Design review of the part built by this model. Coordinates are the model's own, in mm. Face numbers are marked on the shaded views. Coordinates: 2 decimals unless noted, no trailing zeros. Loops run counter-clockwise (first coordinate to the right, second up) from the corner with the lowest first, then second, coordinate; pieces in that order, holes last. Notation, with made-up numbers: (76, -6.75) - (88, -6.75) arc R16 cw to (88, 1.25) - close; hole circle Ø3 at (63.5, 12.25). An arc over 180 degrees is marked (long way). One line per question, with ' | ' between items.
from build123d import *

# Parameters (mm, degrees)
SKETCH1_R               = 6.5
BOSS_EXTRUDE1_DEPTH     = 40
SKETCH2_R               = 7.5
BOSS_EXTRUDE2_DEPTH     = 2
BOSS_EXTRUDE3_DEPTH     = 10
CUT_EXTRUDE1_DEPTH      = 55.004629431
CUT_EXTRUDE1_DEPTH_BACK = 55.004629431
CUT_EXTRUDE2_DEPTH      = 54.619586107
CUT_EXTRUDE2_DEPTH_BACK = 54.619586107
SKETCH5_R               = 0.75
CUT_EXTRUDE3_DEPTH      = 30


with BuildPart() as part:
    # Sketch1 → Boss-Extrude1 (new body)
    with BuildSketch(Plane(origin=(0, 0, 0), x_dir=(0, 0, -1), z_dir=(1, 0, 0))):
        Circle(SKETCH1_R)
    extrude(amount=BOSS_EXTRUDE1_DEPTH)

    # Sketch2 → Boss-Extrude2 (add)
    with BuildSketch(Plane(origin=(40, 0, 0), x_dir=(0, 0, -1), z_dir=(1, 0, 0))):
        Circle(SKETCH2_R)
    extrude(amount=BOSS_EXTRUDE2_DEPTH)

    # Sketch3 → Boss-Extrude3 (add)
    with BuildSketch(Plane(origin=(42, 0, 0), x_dir=(0, 0, -1), z_dir=(1, 0, 0))):
        with BuildLine():
            ThreePointArc((5.590169944, 5), (0, 7.5), (-5.590169944, 5))
            Line((-5.590169944, 5), (-4.898979486, 5))
            Line((-4.898979486, 5), (4.898979486, 5))
            Line((4.898979486, 5), (5.590169944, 5))
        make_face()
        with BuildLine():
            Line((-4.898979486, -5), (-5.590169944, -5))
            ThreePointArc((-5.590169944, -5), (0, -7.5), (5.590169944, -5))
            Line((5.590169944, -5), (4.898979486, -5))
            Line((4.898979486, -5), (-4.898979486, -5))
        make_face()
    extrude(amount=BOSS_EXTRUDE3_DEPTH)

    # Sketch4 → Cut-Extrude1 (cut, two sides: drawn at the far end of the back side and taken through both)
    with BuildSketch(Plane.XZ.offset(-5).offset(-CUT_EXTRUDE1_DEPTH_BACK)):
        with BuildLine():
            Line((42, 5.590169944), (52, 5.590169944))
            Line((52, 5.590169944), (52, -5.590169944))
            Line((52, -5.590169944), (42, -5.590169944))
            Line((42, -5.590169944), (44.640400827, -3.590169944))
            Line((44.640400827, -3.590169944), (47.640400827, -3.590169944))
            add(Edge.make_bspline(
                [(47.640400827, -3.590169944), (50.280133609, -2.393446629), (52.919866391, 0), (50.280133609, 2.393446629), (47.640400827, 3.590169944)],
                knots=[0.178885438, 0.178885438, 0.178885438, 0.178885438, 0.5, 0.821114562, 0.821114562, 0.821114562, 0.821114562], degree=3))
            Line((47.640400827, 3.590169944), (44.640400827, 3.590169944))
            Line((44.640400827, 3.590169944), (42, 5.590169944))
        make_face()
    extrude(amount=CUT_EXTRUDE1_DEPTH + CUT_EXTRUDE1_DEPTH_BACK, mode=Mode.SUBTRACT)

    # Sketch5 → Cut-Extrude2 (cut, two sides: drawn at the far end of the back side and taken through both)
    with BuildSketch(Plane.XZ.offset(-5).offset(-CUT_EXTRUDE2_DEPTH_BACK)):
        with Locations(Location((49, 0, 0), (0, 0, 270))):
            Circle(SKETCH5_R)
    extrude(amount=CUT_EXTRUDE2_DEPTH + CUT_EXTRUDE2_DEPTH_BACK, mode=Mode.SUBTRACT)

    # Sketch6 → Cut-Extrude3 (cut)
    with BuildSketch(Plane.ZY):
        with BuildLine():
            Line((4, -0.5), (4.974937186, -0.5))
            ThreePointArc((4.974937186, -0.5), (3.535533906, -3.535533906), (0.5, -4.974937186))
            Line((0.5, -4.974937186), (0.5, -4))
            Line((0.5, -4), (-0.5, -4))
            Line((-0.5, -4), (-0.5, -4.974937186))
            ThreePointArc((-0.5, -4.974937186), (-3.535533906, -3.535533906), (-4.974937186, -0.5))
            Line((-4.974937186, -0.5), (-4, -0.5))
            Line((-4, -0.5), (-4, 0.5))
            Line((-4, 0.5), (-4.974937186, 0.5))
            ThreePointArc((-4.974937186, 0.5), (-3.535533906, 3.535533906), (-0.5, 4.974937186))
            Line((-0.5, 4.974937186), (-0.5, 4))
            Line((-0.5, 4), (0.5, 4))
            Line((0.5, 4), (0.5, 4.974937186))
            ThreePointArc((0.5, 4.974937186), (3.535533906, 3.535533906), (4.974937186, 0.5))
            Line((4.974937186, 0.5), (4, 0.5))
            Line((4, 0.5), (4, -0.5))
        make_face()
    extrude(amount=-CUT_EXTRUDE3_DEPTH, mode=Mode.SUBTRACT)


solid = part.part
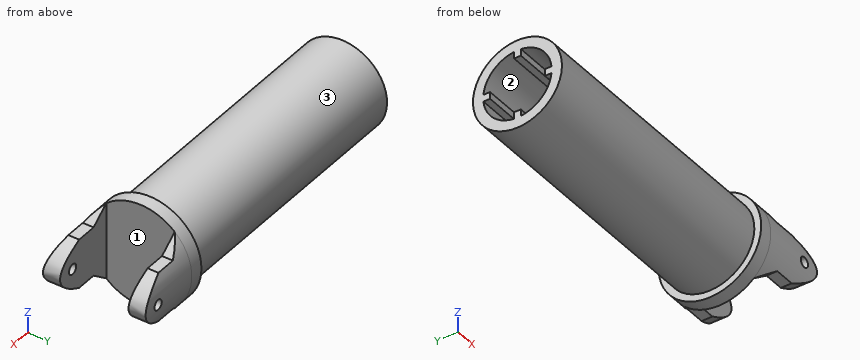
Q1. Take a section at C-C (x = 9). Give the boundary of the cut face in (y, z), plus the area to 3 significant figures.
Returned:
outline: circle Ø13 at (0, 0); hole (-4.97, -0.5) arc R5 ccw to (-0.5, -4.97) - (-0.5, -4) - (0.5, -4) - (0.5, -4.97) arc R5 ccw to (4.97, -0.5) - (4, -0.5) - (4, 0.5) - (4.97, 0.5) arc R5 ccw to (0.5, 4.97) - (0.5, 4) - (-0.5, 4) - (-0.5, 4.97) arc R5 ccw to (-4.97, 0.5) - (-4, 0.5) - (-4, -0.5) - close | area: 58.2 mm²
Q2. To check wall thickness, follow line 1 along X through (y, z) = (5.6, 0); line 2 along X through (y, z) = (6.75, 0); line 3 along X through (y, z) = (-1.75, 4.5). State the ranges of each line that lie inside material, in increasing order.
Returned:
line 1: x = 0 to 48.25, 49.75 to 51.6 | line 2: x = 40 to 48.25, 49.75 to 51.6 | line 3: x = 30 to 42
Q3. Take a section at B-B (y = 0). Give the boundary of the cut face in (x, z), plus the area to 3 significant figures.
Returned:
outline: (0, -6.5) - (40, -6.5) - (40, -7.5) - (42, -7.5) - (42, 7.5) - (40, 7.5) - (40, 6.5) - (0, 6.5) - (0, 4) - (30, 4) - (30, -4) - (0, -4) - close | area: 310 mm²
Q4. Take a section at A-A (x = 43.5). Give the boundary of the cut face in (y, z).
Returned:
outline: (-6.03, -4.45) - (-5, -4.45) - (-5, 4.45) - (-6.03, 4.45) arc R7.5 ccw to start; (5, -4.45) - (6.03, -4.45) arc R7.5 ccw to (6.03, 4.45) - (5, 4.45) - close
Q5. For pin 1 (3 mm diameter, centred on y = -0.5, z = 1, fed in from -X); pin 2 (5 mm diameter, centred on y = 0.5, z = -2, fed in from +X); pin 3 (3 mm diameter, centred on x = 26.5, z = 2, fed in from +Y), all flat-tipped, find the tip position at first contact; note any pin that passes through.
Returned:
pin 1: stops at x = 30 | pin 2: stops at x = 42 | pin 3: stops at y = 6.48
Q6. Draft analysis for pull direction Z (two halves, no side actions). For the marked faces 1, 2 and 3, state which applies: +Z half, -Z half, draft (parallel to the pull), parting line (faces both ways), or undercut.
Returned:
face 1: draft | face 2: undercut | face 3: parting line
Q7. Take a section at D-D (z = 0). State how many separate pieces and enclosed holes the cut face has, plus the area to 4 significant figures.
Returned:
separate pieces: 3 | enclosed holes: 0 | area: 350.5 mm²
